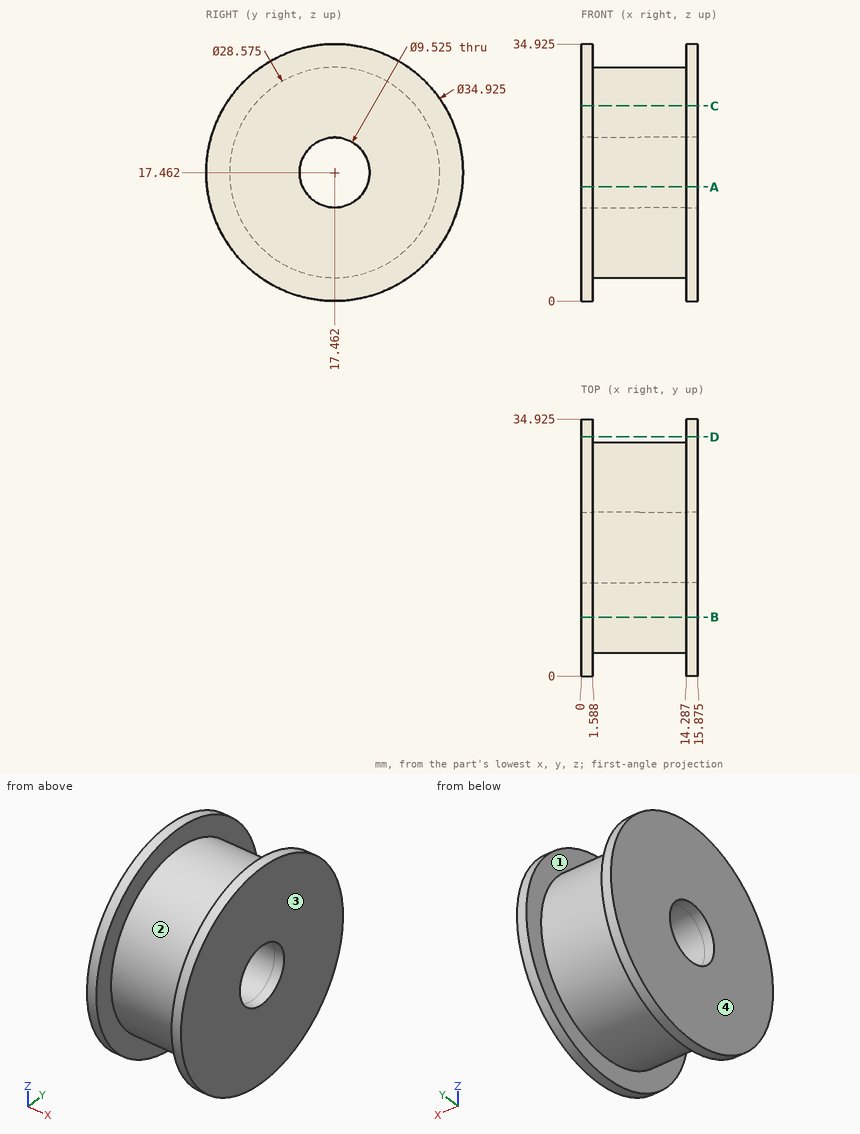
Verification items for this drawing (mm, ordinates from the low corner). Coordinates: 2 decimals unless noted, no trailing zeros. Write each loop counter-clockwise with the first axis right and the second up, starting at its lowest first coordinate (ties: lowest second). Pieces come first, ordered by that corner, then holes. Notation, with made-up numbers: M 52.25,69 L 109.25,69 A15 ccw 109.25,79 Z; hole C 75,-1.75 d7. An arc over 180 degrees is marked long. Answer as a JSON object with one key per item and string values. Group by question number.
(1) Cross-section at D-D, the plane y = 32.5. Record the cut outline in (x, z) (1 decimal).
(2) Cross-section at C-C, the plane z = 26.5. Record the cut outline in (x, y) (1 decimal), and give its area (3 significant figures).
(3) Release check for a two-part mould opening along X. For the marked faces 1, 2, 3 and 4 record: +X half, -X half, draft (parallel to the pull), parting line (faces both ways), or undercut.
(4) Gauge pin test, flat ends, axial feed: pin 1 (5.5 mm diameter, centred on y = 17.46, z = 17.46, fed in from +X); pin 2 (3 mm diameter, centred on x = 9.5, z = 10, fed in from +Y); pin 3 (1.5 mm diameter, centred on x = 7, z = 16.5, fed in from +Y); pin 4 (8 mm diameter, centred on x = 13, y = 5.5, fed in from -Z). Record the tip position at first contact, or that the pin passes through.
(5) Cross-section at A-A, the plane z = 15.5. Record the cut outline in (x, y) (1 decimal).
(6) Material ranges on line 1 (X direction, y = 27, z = 29.5) (1 decimal); line 2 (Z direction, x = 4.75, y = 15) (1 decimal), recorded low to high.
(7) Cross-section at B-B, the plane y = 8. Record the cut outline in (x, z) (1 decimal).
Reply:
{
 "1": {"outline": "M 0,8.6 L 1.6,8.6 L 1.6,26.3 L 0,26.3 Z; M 14.3,8.6 L 15.9,8.6 L 15.9,26.3 L 14.3,26.3 Z"},
 "2": {"outline": "M 0,2.5 L 1.6,2.5 L 1.6,6.4 L 14.3,6.4 L 14.3,2.5 L 15.9,2.5 L 15.9,32.4 L 14.3,32.4 L 14.3,28.5 L 1.6,28.5 L 1.6,32.4 L 0,32.4 Z", "area": "376 mm²"},
 "3": {"face 1": "undercut", "face 2": "undercut", "face 3": "+X half", "face 4": "-X half"},
 "4": {"pin 1": "through", "pin 2": "y = 30.45", "pin 3": "y = 31.75", "pin 4": "z = 2.03"},
 "5": {"outline": "M 0,0.1 L 1.6,0.1 L 1.6,3.3 L 14.3,3.3 L 14.3,0.1 L 15.9,0.1 L 15.9,13.1 L 0,13.1 Z; M 0,21.8 L 15.9,21.8 L 15.9,34.8 L 14.3,34.8 L 14.3,31.6 L 1.6,31.6 L 1.6,34.8 L 0,34.8 Z"},
 "6": {"line 1": "0 to 1.6, 14.3 to 15.9", "line 2": "3.4 to 13.4, 21.5 to 31.5"},
 "7": {"outline": "M 0,2.8 L 1.6,2.8 L 1.6,6.8 L 14.3,6.8 L 14.3,2.8 L 15.9,2.8 L 15.9,32.1 L 14.3,32.1 L 14.3,28.2 L 1.6,28.2 L 1.6,32.1 L 0,32.1 Z"}
}
